from build123d import *

# Parameters (mm, degrees)
F0_W     = 50.984893
F0_H     = 2.100501
F0_W_2   = 50.602986
F0_H_2   = 2.482414
F0_W_3   = 51.175848
F0_H_3   = 2.86432
F0_H_4   = 3.246229
F0_W_4   = 50.412029
F0_W_5   = 50.221075
F0_W_6   = 50.030118
F0_H_5   = 2.673368
F0_W_7   = 49.839167
F0_H_6   = 2.864324
F0_W_8   = 49.731534
F0_H_7   = 2.725012
F0_W_9   = 50.639872
F0_H_8   = 2.49793
F1_DEPTH = 5


with BuildPart() as f1:
    # F0 (on Front) → F1 (new body)
    with BuildSketch(Plane.XZ):
        Polygon((-48.025098, -52.537646), (-48.025098, -55.854235), (47.834139, -55.854235), (47.834139, -52.537646), (12.798216, -52.537646), (12.798216, -50.039716), (47.834139, -50.039716), (47.834139, -41.532639), (12.698486, -41.532639), (12.698486, -38.859274), (47.834139, -38.859274), (47.834139, -29.120585), (12.698486, -29.120585), (12.698486, -26.06531), (47.834139, -26.06531), (47.834139, -16.326623), (12.125621, -16.326623), (12.125621, -12.889439), (47.834139, -12.889439), (47.834139, -3.91457), (12.125621, -3.91457), (12.125621, -1.43216), (47.834139, -1.43216), (47.834139, 8.497482), (12.125621, 8.497482), (12.125621, 11.552757), (47.834139, 11.552757), (47.834139, 20.71858), (12.125621, 20.71858), (12.125621, 23.5829), (47.834139, 23.5829), (47.834139, 31.030132), (12.125621, 31.030132), (12.125621, 33.703495), (47.834139, 33.703495), (47.834139, 41.475393), (12.116962, 41.475393), (12.116962, 44.200405), (47.834139, 44.200405), (47.834139, 51.240031), (12.125621, 51.240031), (12.125621, 53.510878), (47.834139, 53.510878), (47.834139, 60.5505), (12.344047, 60.5505), (12.344047, 63.502602), (47.834139, 63.502602), (47.834139, 66.356741), (-48.025098, 66.356741), (-48.025098, 63.275516), (-11.49984, 63.275516), (-11.49984, 60.5505), (-48.025098, 60.5505), (-48.025098, 53.510878), (-11.49984, 53.510878), (-11.49984, 51.012948), (-48.025098, 51.012948), (-48.025098, 43.973323), (-11.726924, 43.973323), (-11.726924, 41.021224), (-48.025098, 41.021224), (-48.025098, 33.703495), (-11.361802, 33.703495), (-11.361802, 30.457268), (-48.025098, 30.457268), (-48.025098, 22.819081), (-11.361802, 22.819081), (-11.361802, 19.763807), (-48.025098, 19.763807), (-48.025098, 10.979893), (-11.361802, 10.979893), (-11.361802, 7.924618), (-48.025098, 7.924618), (-48.025098, -1.43216), (-11.361802, -1.43216), (-11.361802, -4.29648), (-48.025098, -4.29648), (-48.025098, -12.889439), (-11.361802, -12.889439), (-11.361802, -16.326623), (-48.025098, -16.326623), (-48.025098, -26.06531), (-11.170847, -26.06531), (-11.170847, -29.120585), (-48.025098, -29.120585), (-48.025098, -38.859274), (-11.170847, -38.859274), (-11.170847, -41.532639), (-48.025098, -41.532639), (-48.025098, -50.039716), (-11.272755, -50.039716), (-11.272755, -52.537646), align=None)
        with Locations((2.291455, -46.783892)):
            Rectangle(F0_W, F0_H, mode=Mode.SUBTRACT)
        with Locations((2.100502, -33.989929)):
            Rectangle(F0_W_2, F0_H_2, mode=Mode.SUBTRACT)
        with Locations((2.386933, -21.195967)):
            Rectangle(F0_W_3, F0_H_3, mode=Mode.SUBTRACT)
        with Locations((2.291455, -8.592959)):
            Rectangle(F0_W, F0_H_4, mode=Mode.SUBTRACT)
        with Locations((2.005024, 3.437183)):
            Rectangle(F0_W_4, F0_H_4, mode=Mode.SUBTRACT)
        with Locations((1.909546, 15.276373)):
            Rectangle(F0_W_5, F0_H_4, mode=Mode.SUBTRACT)
        with Locations((1.814068, 27.401994)):
            Rectangle(F0_W_6, F0_H_5, mode=Mode.SUBTRACT)
        with Locations((1.718592, 37.236158)):
            Rectangle(F0_W_7, F0_H_6, mode=Mode.SUBTRACT)
        with Locations((1.557527, 47.606677)):
            Rectangle(F0_W_8, F0_H_7, mode=Mode.SUBTRACT)
        with Locations((2.011696, 56.803601)):
            Rectangle(F0_W_9, F0_H_8, mode=Mode.SUBTRACT)
    extrude(amount=F1_DEPTH)


solid = f1.part
The model under review builds one solid part; all positions refer to its coordinate system, in mm. A direction names the side the tool comes from. Round coordinates to 2 decimals unless told otherwise and drop trailing zeros. Write item = value, one per line. Start each with the question number.
Item 1: To check wall thickness, follow L1, parallel to X at y = -3.1, z = -46; L2, parallel to X at y = -4.35, z = 58; L3, parallel to X at y = -0.5, z = -29. State the ranges of each line that lie inside material, in increasing order.
Item 2: Take a section at A-A on x = -4.5. Count the separate pieces of the cut face and the enclosed holes in it, plus the area to 3 significant figures.
Item 3: For faces 4 (the flat face through (2, -2, -19.764)), 5 (the flat face through (-48.025, -2, 57)), 6 (the flat face through (-11.171, -2, -40)), 7 (the flat face through (12.126, -2, 22)), list the 3-axis set-ups (+Z, -Z, +X, -X, +Y, -Y) from which the entire face can be reached by the end or side of a thin tool; tool diameter is ignored.
Item 4: Insertion check: pin 1 (1.5 mm diameter, centred on y = -3.5, z = 21, fed in from -X). The pin has a flat end and moves straight along its axis. Give the tip position at first contact, or say it passes through.
Item 5: Mouldability with a two-part tool opening along X and no side actions: class faces 1 (the flat face through (30, -2, 23.583)), 2 (the flat face through (27.02, -2, 15)), 3 (the flat face through (-11.5, -2, 62)) as released by +X, released by -X, zero draft, split by the parting line, or undercut.
Result:
q1.L1 = -48.03 to -23.2, 27.78 to 47.83
q1.L2 = -48.03 to -23.31, 27.33 to 47.83
q1.L3 = -11.17 to 12.7
q2.separate_pieces = 11
q2.enclosed_holes = 0
q2.area = 471 mm²
q3.face_4 = +Y, -Y
q3.face_5 = +Z, -Z, -X, +Y, -Y
q3.face_6 = -X, +Y, -Y
q3.face_7 = +X, +Y, -Y
q4.pin_1 = -11.36
q5.face_1 = zero draft
q5.face_2 = undercut
q5.face_3 = released by -X
